```python
from build123d import *

# Parameters (mm, degrees)
SALIENTE_EXTRUIR1_DEPTH = 1.6002
PINOUT_R                = 0.254
CORTAR_EXTRUIR2_DEPTH   = 1.6002
DRILLS_R                = 1.5875
CORTAR_EXTRUIR3_DEPTH   = 1.6002


with BuildPart() as part:
    # Board → Saliente-Extruir1 (new body)
    with BuildSketch(Plane(origin=(0, 0, 0), x_dir=(1, 0, 0), z_dir=(0, 1, 0))):
        Polygon((57.12, 37.846), (57.12, 5.08), (54.64, 2.54), (54.64, 0), (0, 0), (0, 53.378473106), (53.075207648, 53.378473106), (54.64, 51.813680753), (54.64, 40.386), align=None)
    extrude(amount=SALIENTE_EXTRUIR1_DEPTH)

    # Pinout → Cortar-Extruir2 (cut)
    with BuildSketch(Plane(origin=(0, 0, 0), x_dir=(1, 0, 0), z_dir=(0, 1, 0))):
        with Locations(Location((52.07000008, 2.54, 0), (0, 0, 270))):
            Circle(PINOUT_R)
        with Locations(Location((49.53000008, 2.54, 0), (0, 0, 270))):
            Circle(PINOUT_R)
        with Locations(Location((46.99000008, 2.54, 0), (0, 0, 270))):
            Circle(PINOUT_R)
        with Locations(Location((44.45000008, 2.54, 0), (0, 0, 270))):
            Circle(PINOUT_R)
        with Locations(Location((41.91000008, 2.54, 0), (0, 0, 270))):
            Circle(PINOUT_R)
        with Locations(Location((39.37000008, 2.54, 0), (0, 0, 270))):
            Circle(PINOUT_R)
        with Locations(Location((34.29000008, 2.54, 0), (0, 0, 270))):
            Circle(PINOUT_R)
        with Locations(Location((31.75000008, 2.54, 0), (0, 0, 270))):
            Circle(PINOUT_R)
        with Locations(Location((29.21000008, 2.54, 0), (0, 0, 270))):
            Circle(PINOUT_R)
        with Locations(Location((26.67000008, 2.54, 0), (0, 0, 270))):
            Circle(PINOUT_R)
        with Locations(Location((24.13000008, 2.54, 0), (0, 0, 270))):
            Circle(PINOUT_R)
        with Locations(Location((21.59000008, 2.54, 0), (0, 0, 270))):
            Circle(PINOUT_R)
        with Locations(Location((19.05000008, 2.54, 0), (0, 0, 270))):
            Circle(PINOUT_R)
        with Locations(Location((16.51000008, 2.54, 0), (0, 0, 270))):
            Circle(PINOUT_R)
        with Locations(Location((52.07000008, 50.8, 0), (0, 0, 270))):
            Circle(PINOUT_R)
        with Locations(Location((49.53000008, 50.8, 0), (0, 0, 270))):
            Circle(PINOUT_R)
        with Locations(Location((46.99000008, 50.8, 0), (0, 0, 270))):
            Circle(PINOUT_R)
        with Locations(Location((44.45000008, 50.8, 0), (0, 0, 270))):
            Circle(PINOUT_R)
        with Locations(Location((41.91000008, 50.8, 0), (0, 0, 270))):
            Circle(PINOUT_R)
        with Locations(Location((39.37000008, 50.8, 0), (0, 0, 270))):
            Circle(PINOUT_R)
        with Locations(Location((36.83000008, 50.8, 0), (0, 0, 270))):
            Circle(PINOUT_R)
        with Locations(Location((34.29000008, 50.8, 0), (0, 0, 270))):
            Circle(PINOUT_R)
        with Locations(Location((30.25600002, 50.8, 0), (0, 0, 270))):
            Circle(PINOUT_R)
        with Locations(Location((27.71600002, 50.8, 0), (0, 0, 270))):
            Circle(PINOUT_R)
        with Locations(Location((25.17600002, 50.8, 0), (0, 0, 270))):
            Circle(PINOUT_R)
        with Locations(Location((22.63600002, 50.8, 0), (0, 0, 270))):
            Circle(PINOUT_R)
        with Locations(Location((20.09600002, 50.8, 0), (0, 0, 270))):
            Circle(PINOUT_R)
        with Locations(Location((17.55600002, 50.8, 0), (0, 0, 270))):
            Circle(PINOUT_R)
        with Locations(Location((15.01600002, 50.8, 0), (0, 0, 270))):
            Circle(PINOUT_R)
        with Locations(Location((12.47600002, 50.8, 0), (0, 0, 270))):
            Circle(PINOUT_R)
        with Locations(Location((9.93600002, 50.8, 0), (0, 0, 270))):
            Circle(PINOUT_R)
        with Locations(Location((7.39600002, 50.8, 0), (0, 0, 270))):
            Circle(PINOUT_R)
    extrude(amount=CORTAR_EXTRUIR2_DEPTH, mode=Mode.SUBTRACT)

    # Drills → Cortar-Extruir3 (cut)
    with BuildSketch(Plane(origin=(0, 0, 0), x_dir=(1, 0, 0), z_dir=(0, 1, 0))):
        with Locations(Location((3.84, 50.8, 0), (0, 0, 270))):
            Circle(DRILLS_R)
        with Locations(Location((54.64, 35.56, 0), (0, 0, 270))):
            Circle(DRILLS_R)
        with Locations(Location((54.64, 7.62, 0), (0, 0, 270))):
            Circle(DRILLS_R)
        with Locations(Location((2.540000009, 2.54, 0), (0, 0, 270))):
            Circle(DRILLS_R)
    extrude(amount=CORTAR_EXTRUIR3_DEPTH, mode=Mode.SUBTRACT)


solid = part.part
```
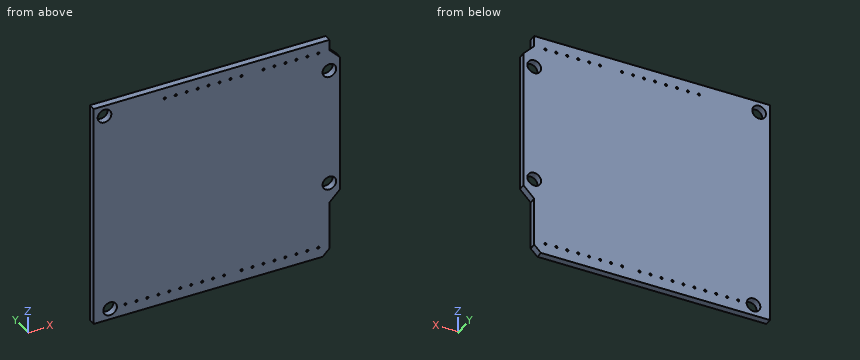
Model file for the job. Use its own axes, mm. Give positions to 0.01 mm unless a question says otherwise; leave off trailing zeros. Loops run counter-clockwise (first coordinate to the right, second up) from the corner with the lowest first, then second, coordinate; pieces in that order, holes last. Notation, with made-up numbers: (-10, -6.75) - (23, -6.75) arc R33 ccw to (23, 27.25) - close; hole circle Ø11 at (36.5, 58). An arc over 180 degrees is marked (long way). One line per item, written item: value. Start each with the question number.
1. Probe L1, parallel to Z at x = 44.5, y = 1.4; L2, parallel to X at y = 1, z = -9; L3, parallel to Z at x = 34.5, y = 0.65. List the from-to ranges inside material, lowest first. Write a range as from..to.
2. Slice it at C-C (y = 0.5). Give the number of separate pieces and of enclosed holes in the cut face, plus the area to 3 significant figures.
3. Slice it at B-B (z = -7.62). List the corners of the cut face in (x, y).
4. Slice it at A-A (z = -35). List the corners of the cut face in (x, y).
5. Pin check, flat tips, straight feed: pin 1 (0.8 mm diameter, centred on y = 0.5, z = -1, fed in from +X); pin 2 (3.5 mm diameter, centred on x = 2.54, z = -2.54, fed in from +Y). Stop position of each tip, or through.
Solution:
1. L1: z = -53.38..-51.05, -50.55..-2.79, -2.29..0
1. L2: x = 0..53.86, 55.42..57.12
1. L3: z = -53.38..-50.94, -50.66..-2.68, -2.4..0
2. separate pieces: 1
2. enclosed holes: 36
2. area: 2,960 mm^2
3. outline: (0, 0) - (53.05, 0) - (53.05, 1.6) - (0, 1.6) - close; (56.23, 0) - (57.12, 0) - (57.12, 1.6) - (56.23, 1.6) - close
4. outline: (0, 0) - (53.15, 0) - (53.15, 1.6) - (0, 1.6) - close; (56.13, 0) - (57.12, 0) - (57.12, 1.6) - (56.13, 1.6) - close
5. pin 1: stops at x = 54.64
5. pin 2: stops at y = 1.6
